from build123d import *

# Parameters (mm, degrees)
SKETCH1_W                            = 47.625
SKETCH1_H                            = 352.425
BASE_FLANGE1_DEPTH                   = 3.175
EDGE_FLANGE1_STRIP_W                 = 18.7
EDGE_FLANGE1_STRIP_H                 = 3.175
EDGE_FLANGE1_STRIP_CUT_DEPTH         = 352.425
EDGE_FLANGE1_DEPTH                   = 352.425
EDGE_FLANGE2_STRIP_W                 = 18.7
EDGE_FLANGE2_STRIP_H                 = 3.175
EDGE_FLANGE2_STRIP_CUT_DEPTH         = 352.425
EDGE_FLANGE2_DEPTH                   = 352.425
BOSS_EXTRUDE1_DEPTH                  = 3.175
BOSS_EXTRUDE2_DEPTH                  = 3.175
F_17_64_START                        = -3.175
F_17_64_0_26563_DIAMETER_SLOT1_DEPTH = 53.975
F_17_64_0_26563_DIAMETER_HOLE2_D     = 6.747002
SKETCH21_W                           = 9.525
SKETCH21_H                           = 9.525
CUT_EXTRUDE1_DEPTH                   = 392.259979106
EDGE_FLANGE5_STRIP_W                 = 18.7
EDGE_FLANGE5_STRIP_H                 = 3.175
EDGE_FLANGE5_STRIP_CUT_DEPTH         = 63.5
EDGE_FLANGE5_RELIEF_W                = 20.2875
EDGE_FLANGE5_RELIEF_H                = 1.5875
EDGE_FLANGE5_RELIEF_CUT_DEPTH        = 3.175
EDGE_FLANGE5_DEPTH                   = 63.5
FILLET2_R                            = 6.35
F_17_64_0_26563_DIAMETER_HOLE3_D     = 6.747002
FILLET3_R                            = 3.175
CUT_EXTRUDE3_DEPTH                   = 395.939882292
CUT_EXTRUDE3_DEPTH_BACK              = 395.939882292
SKETCH30_W                           = 3.175
SKETCH30_H                           = 28.575
FILLET4_R                            = 3.175


# Read off the part's stored shape, not the designer's step: 17/64 (0.26563) Diameter Slot1
# Sheet-metal steps are written as plain solids
with BuildPart() as part:
    # Sketch1 → Base-Flange1 (new body)
    with BuildSketch(Plane(origin=(0, 0, 0), x_dir=(1, 0, 0), z_dir=(0, 1, 0))):
        with Locations((23.8125, 176.2125)):
            Rectangle(SKETCH1_W, SKETCH1_H)
    extrude(amount=-BASE_FLANGE1_DEPTH)

    # Edge-Flange1 strip (across the edge) → Edge-Flange1 strip cut (cut)
    with BuildSketch(Plane(origin=(47.625, -3.175, -352.425), x_dir=(-1, 0, 0), z_dir=(0, 0, 1))):
        with Locations((-6.35, -1.5875)):
            Rectangle(EDGE_FLANGE1_STRIP_W, EDGE_FLANGE1_STRIP_H)
    extrude(amount=EDGE_FLANGE1_STRIP_CUT_DEPTH, mode=Mode.SUBTRACT)

    # Edge-Flange1 section (across the edge) → Edge-Flange1 (add)
    with BuildSketch(Plane(origin=(47.625, -3.175, -352.425), x_dir=(-1, 0, 0), z_dir=(0, 0, 1))):
        with BuildLine():
            Line((-3.175, 3), (-3.175, 34.925))
            Line((-3.175, 34.925), (0, 34.925))
            Line((0, 34.925), (0, 3))
            ThreePointArc((0, 3), (0.878679656, 0.878679656), (3, 0))
            Line((3, 0), (3, -3.175))
            ThreePointArc((3, -3.175), (-1.366384374, -1.366384374), (-3.175, 3))
        make_face()
    extrude(amount=EDGE_FLANGE1_DEPTH)

    # Edge-Flange2 strip (across the edge) → Edge-Flange2 strip cut (cut)
    with BuildSketch(Plane(origin=(0, -3.175, 0), x_dir=(1, 0, 0), z_dir=(0, 0, -1))):
        with Locations((-6.35, -1.5875)):
            Rectangle(EDGE_FLANGE2_STRIP_W, EDGE_FLANGE2_STRIP_H)
    extrude(amount=EDGE_FLANGE2_STRIP_CUT_DEPTH, mode=Mode.SUBTRACT)

    # Edge-Flange2 section (across the edge) → Edge-Flange2 (add)
    with BuildSketch(Plane(origin=(0, -3.175, 0), x_dir=(1, 0, 0), z_dir=(0, 0, -1))):
        with BuildLine():
            Line((-3.175, 3), (-3.175, 34.925))
            Line((-3.175, 34.925), (0, 34.925))
            Line((0, 34.925), (0, 3))
            ThreePointArc((0, 3), (0.878679656, 0.878679656), (3, 0))
            Line((3, 0), (3, -3.175))
            ThreePointArc((3, -3.175), (-1.366384374, -1.366384374), (-3.175, 3))
        make_face()
    extrude(amount=EDGE_FLANGE2_DEPTH)

    # Sketch12 → Boss-Extrude1 (add)
    with BuildSketch(Plane.ZY.offset(3.175)):
        Polygon((-384.175, -50.8), (-384.175, -25.4), (-352.425, -15.875), (-352.425, -38.1), (-314.325, -38.1), (-356.658333333, -50.8), align=None)
    extrude(amount=-BOSS_EXTRUDE1_DEPTH)

    # Sketch13 → Boss-Extrude2 (add)
    with BuildSketch(Plane(origin=(50.8, 0, 0), x_dir=(0, 0, -1), z_dir=(1, 0, 0))):
        Polygon((352.425, -15.875), (352.425, -38.1), (314.325, -38.1), (356.658333333, -50.8), (384.175, -50.8), (384.175, -25.4), align=None)
    extrude(amount=-BOSS_EXTRUDE2_DEPTH)

    # 17/64 (0.26563) Diameter Slot1 outline → 17/64 (0.26563) Diameter Slot1 (cut)
    with BuildSketch(Plane.YZ.offset(F_17_64_START)):
        with BuildLine():
            ThreePointArc((-41.473501, -377.626499), (-38.1, -381), (-34.726499, -377.626499))
            Line((-34.726499, -377.626499), (-34.726499, -371.673501))
            ThreePointArc((-34.726499, -371.673501), (-38.1, -368.3), (-41.473501, -371.673501))
            Line((-41.473501, -371.673501), (-41.473501, -377.626499))
        make_face()
    extrude(amount=F_17_64_0_26563_DIAMETER_SLOT1_DEPTH, mode=Mode.SUBTRACT)

    # 17/64 (0.26563) Diameter Hole2 (through all)
    with Locations(Plane(origin=(0, 0, 0), x_dir=(1, 0, 0), z_dir=(0, 1, 0))):
        with Locations((23.8125, 22.225), (23.8125, 60.325)):
            Hole(F_17_64_0_26563_DIAMETER_HOLE2_D / 2)

    # Sketch21 → Cut-Extrude1 (cut, through all)
    with BuildSketch(Plane.ZY.offset(3.175)):
        with Locations((-4.7625, -33.3375)):
            Rectangle(SKETCH21_W, SKETCH21_H)
    extrude(amount=-CUT_EXTRUDE1_DEPTH, mode=Mode.SUBTRACT)

    # Edge-Flange5 strip (across the edge) → Edge-Flange5 strip cut (cut)
    with BuildSketch(Plane(origin=(-3.175, -38.1, -73.025), x_dir=(0, 1, 0), z_dir=(0, 0, 1))):
        with Locations((-3.175, -1.5875)):
            Rectangle(EDGE_FLANGE5_STRIP_W, EDGE_FLANGE5_STRIP_H)
    edge_flange5_strip_cut = extrude(amount=EDGE_FLANGE5_STRIP_CUT_DEPTH, mode=Mode.SUBTRACT)

    # Edge-Flange5 relief (on the sheet) → Edge-Flange5 relief cut (cut)
    with BuildSketch(Plane(origin=(-3.175, -31.925, -73.025), x_dir=(0, 1, 0), z_dir=(-1, 0, 0))):
        with Locations((-8.55625, 0.79375)):
            Rectangle(EDGE_FLANGE5_RELIEF_W, EDGE_FLANGE5_RELIEF_H)
    edge_flange5_relief_cut = extrude(amount=-EDGE_FLANGE5_RELIEF_CUT_DEPTH, mode=Mode.SUBTRACT)

    # Edge-Flange5 section (across the edge) → Edge-Flange5 (add)
    with BuildSketch(Plane(origin=(-3.175, -38.1, -73.025), x_dir=(0, 1, 0), z_dir=(0, 0, 1))):
        with BuildLine():
            Line((0, 3), (0, 22.225))
            Line((0, 22.225), (3.175, 22.225))
            Line((3.175, 22.225), (3.175, 3))
            ThreePointArc((3.175, 3), (4.053679656, 0.878679656), (6.175, 0))
            Line((6.175, 0), (6.175, -3.175))
            ThreePointArc((6.175, -3.175), (1.808615626, -1.366384374), (0, 3))
        make_face()
    edge_flange5 = extrude(amount=EDGE_FLANGE5_DEPTH)

    # Fillet2
    fillet2_edges = [part.edges().sort_by_distance(p)[0] for p in [
        (-1.5875, -38.1, -314.325),
        (-1.5875, -50.8, -356.658333333),
        (-1.5875, -50.8, -384.175),
        (-1.5875, -25.4, -384.175),
        (-1.5875, -15.875, -352.425),
        (49.2125, -38.1, -314.325),
        (49.2125, -15.875, -352.425),
        (49.2125, -25.4, -384.175),
        (49.2125, -50.8, -384.175),
        (49.2125, -50.8, -356.658333333),
    ]]
    fillet(fillet2_edges, radius=FILLET2_R)

    # Mirror1: Edge-Flange5 strip cut, Edge-Flange5 relief cut, Edge-Flange5 across plane
    add(edge_flange5_strip_cut.mirror(Plane.ZY.offset(-23.8125)), mode=Mode.SUBTRACT)
    add(edge_flange5_relief_cut.mirror(Plane.ZY.offset(-23.8125)), mode=Mode.SUBTRACT)
    add(edge_flange5.mirror(Plane.ZY.offset(-23.8125)))

    # 17/64 (0.26563) Diameter Hole3 (through all)
    with Locations(Plane(origin=(0, -34.925, 0), x_dir=(1, 0, 0), z_dir=(0, 1, 0))):
        with Locations((-15.875, 60.325), (-15.875, 22.225)):
            f_17_64_0_26563_diameter_hole3 = Hole(F_17_64_0_26563_DIAMETER_HOLE3_D / 2)

    # Mirror2: 17/64 (0.26563) Diameter Hole3 across plane
    add(f_17_64_0_26563_diameter_hole3.mirror(Plane.ZY.offset(-23.8125)), mode=Mode.SUBTRACT)

    # Fillet3
    fillet3_edges = [part.edges().sort_by_distance(p)[0] for p in [
        (-25.4, -36.5125, -73.025),
        (-25.4, -36.5125, -9.525),
        (73.025, -36.5125, -9.525),
        (73.025, -36.5125, -73.025),
    ]]
    fillet(fillet3_edges, radius=FILLET3_R)

    # Sketch30 → Cut-Extrude3 (cut, two sides: drawn at the far end of the back side and taken through both)
    with BuildSketch(Plane.ZY.offset(3.175).offset(-CUT_EXTRUDE3_DEPTH_BACK)):
        with Locations((-1.5875, -14.2875)):
            Rectangle(SKETCH30_W, SKETCH30_H)
    extrude(amount=CUT_EXTRUDE3_DEPTH + CUT_EXTRUDE3_DEPTH_BACK, mode=Mode.SUBTRACT)

    # Fillet4
    fillet4_edges = [part.edges().sort_by_distance(p)[0] for p in [
        (49.2125, -28.575, -3.175),
        (-1.5875, -28.575, -3.175),
    ]]
    fillet(fillet4_edges, radius=FILLET4_R)


solid = part.part
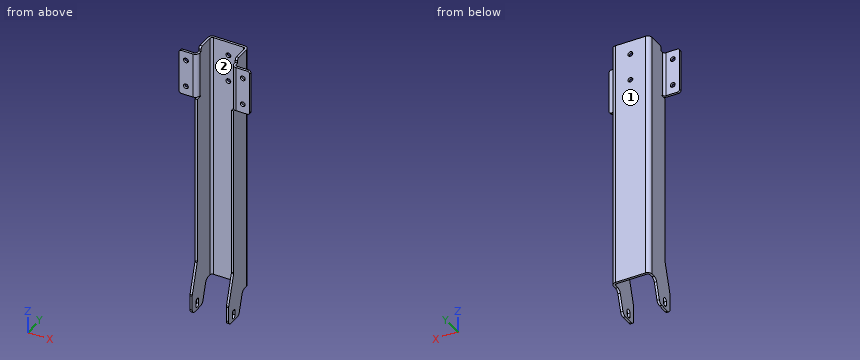
Can you work these out from the model? Positions are in its coordinate system, mm. Face numbers are marked on the shaded views. Coordinates: 2 decimals unless noted, no trailing zeros. Write each loop counter-clockwise with the first axis right and the second up, starting at its lowest first coordinate (ties: lowest second). Pieces come first, ordered by that corner, then holes. Notation, with made-up numbers: M -28.5,66 L -14.5,66 A24 cw -14.5,105 Z; hole C -38.5,9.25 d4. An arc over 180 degrees is marked long. Use one line per item in the form item = value.
Q1. If we section it at B-B (z = -145.5): Write out the boundary of the cut face in (x, y) (3 decimals).
Model answer:
outline = M -3.175,-38.1 L 0,-38.1 L 0,-6.175 A3 cw 3,-3.175 L 44.625,-3.175 A3 cw 47.625,-6.175 L 47.625,-38.1 L 50.8,-38.1 L 50.8,-6.175 A6.175 ccw 44.625,0 L 3,0 A6.175 ccw -3.175,-6.175 Z
Q2. If we section it at C-C (x = 16.5): Write out the boundary of the cut face in (y, z) (3 decimals).
Model answer:
outline = M -3.175,-352.425 L 0,-352.425 L 0,-3.175 L -3.175,-3.175 Z
Q3. For P1, Ø1.3, axis at x = 49, z = -73.5, coming from the -Y side; P2, Ø1.5, axis at y = -27, z = -298.5, coming from the -X side (3 decimals); P3, Ø6, axis at x = -11, z = -30.5, coming from the +Y side (3 decimals), each with a flat end and sliding along its axis, tell me the tip position at first contact or that it passes through.
Model answer:
P1 = -36.3
P2 = -3.175
P3 = -34.925
Q4. We'd pull the mould along X, two halves only. Please class the marked faces 1 and 2: +X half, -X half, draft (parallel to the pull), parting line (faces both ways), or undercut.
Model answer:
face_1 = draft
face_2 = undercut
Q5. I need wall thicknesses on line 1 along Z through (x, y) = (63, -37) (3 decimals); line 2 along X through (y, z) = (-18.5, -322.5) (3 decimals); line 3 along Y through (x, z) = (26, -179) (3 decimals). Which ranges of each line are inside material? Lowest first, please. Write a range as from..to.
Model answer:
line_1 = -73.025..-63.661, -56.989..-25.561, -18.889..-9.525
line_2 = -3.175..0, 47.625..50.8
line_3 = -3.175..0
Q6. If we section it at A-A (x = 63.5): Write out the boundary of the cut face in (y, z) (1 decimal), then the cut area to 3 significant figures.
Model answer:
outline = M -38.1,-73 L -34.9,-73 L -34.9,-63.7 L -38.1,-63.7 Z; M -38.1,-57 L -34.9,-57 L -34.9,-25.6 L -38.1,-25.6 Z; M -38.1,-18.9 L -34.9,-18.9 L -34.9,-9.5 L -38.1,-9.5 Z
area = 159 mm^2
